Autodesk Inventor part; units mm, degrees
ref_plane "YZ Plane" through (0, 0, 0) normal (1, 0, 0) x (0, 1, 0)
ref_plane "XZ Plane" through (0, 0, 0) normal (0, 1, 0) x (-1, 0, 0)
ref_plane "XY Plane" through (0, 0, 0) normal (0, 0, 1) x (1, 0, 0)
sketch "Эскиз1" plane through (0, 0, 0) normal (0, 0, 1) x (1, 0, 0)
  circle A0 centre (0, 0) radius 11.3
  circle A1 centre (-7.7068, -2.1459) radius 1.55
  circle A2 centre (1.995, 7.7473) radius 1.55
  circle A3 centre (-7.7068, -2.1459) radius 1.55
  circle A4 centre (1.995, 7.7473) radius 1.55
  circle A5 centre (5.7118, -5.6014) radius 1.55
  circle A6 centre (0, 0) radius 11.3
  circle A7 centre (7.7568, 1.9574) radius 2
  circle A8 centre (-2.1832, -7.6963) radius 2
  circle A9 centre (-5.5736, 5.7389) radius 2
  circle A10 centre (0, 0) radius 11.1
  point P0 (0, 0)
extrude "Выдавливание1" add sketch "Эскиз1" along normal blind 5 contours A7 | A8 | A9 | A10
sketch "Эскиз2" plane through (0, 0, 0) normal (0, 0, -1) x (-1, 0, 0)
  circle A0 centre (5.5736, 5.7389) radius 2
  circle A1 centre (2.1832, -7.6963) radius 2
  circle A2 centre (-7.7568, 1.9574) radius 2
  circle A3 centre (5.5736, 5.7389) radius 1.9
  circle A4 centre (2.1832, -7.6963) radius 1.9
  circle A5 centre (-7.7568, 1.9574) radius 1.9
  point P0 (0, 0)
  dimension "d3" = 0.1
  dimension "d4" = 0.1
  dimension "d5" = 0.1
extrude "Выдавливание2" add sketch "Эскиз2" along normal blind 5 contours A3 | A4 | A5
chamfer "Фаска1" distance 1 angle 45 6 edges at (9.6568, 1.9574, -5) (-3.6736, 5.7389, -5) (-0.2832, -7.6963, -5) (4.1618, -5.6014, 5) (0.445, 7.7473, 5) (-9.2568, -2.1459, 5)
properties part number "ВедущееКолесоВнутр"
Model file for the job. Use its own axes, mm. A direction names the side the tool comes from. Coordinates: 2 decimals unless noted, no trailing zeros. Write each loop counter-clockwise with the first axis right and the second up, starting at its lowest first coordinate (ties: lowest second). Pieces come first, ordered by that corner, then holes. Notation, with made-up numbers: (-24, 76) - (16, 76) arc R38 ccw to (16, 114) - close; hole circle Ø10 at (26, 58.5). An arc over 180 degrees is marked (long way). Write each question's results on one line, items separated by ' | '. Start each with the question number.
1) Flat gauge pins, fed straight in: P1, Ø1.5, axis at x = 8.5, z = 1.5, coming from the +Y side; P2, Ø3, axis at y = -7.5, z = 0, coming from the +X side; P3, Ø6, axis at x = 7.5, y = -9, coming from the -Z side; P4, Ø8, axis at x = 7.5, y = -5, coming from the +Z side. Where does each tip first touch, or does it go through?
2) Mould opens along X. For faces 1 (the face through (6.43, -4.23, 1.97)), 2 (the face through (-3.06, -6.01, -1.97)), 3 (the face through (-6, 6, -5)) say: pulls with the +X half, pulls with the -X half, needs draft (parallel to the pull), parting line crosses it, or undercut.
3) 3-axis set-ups, long thin cutter, end or side, ignore diameter. For faces 4 (the face through (-4.173, 4.455, -1.972)), 5 (the face through (-2, -8, -5)): which of +Z, -Z, +X, -X, +Y, -Y reach the whole face in a straight line?
4) Cut at A-A (z = 2.25). Write the cut outline in (x, y) (3 decimals), then the cut area to 3 significant figures.
5) Probe line 1 along Y through (x, z) = (-0.25, 1.75); line 2 along Z through (x, y) = (-4.5, 3.25); line 3 along Y through (x, z) = (-7.25, -2). List the from-to ranges inside material, lowest first. Write a range as from..to.
6) Cut at B-B (z = -0.75). Write the cut outline in (x, y), then the cut area to 3 significant figures.
Returned:
1) P1: y = 7.95 | P2: x = 9.34 | P3: z = 0 | P4: z = 5
2) face 1: undercut | face 2: parting line crosses it | face 3: needs draft
3) face 4: -Z | face 5: -Z, +X, -X, +Y, -Y
4) outline: circle Ø22.2 at (0, 0); hole circle Ø3.1 at (-7.707, -2.146); hole circle Ø3.1 at (1.995, 7.747); hole circle Ø3.1 at (5.712, -5.601) | area: 364 mm^2
5) line 1: -11.1..11.1 | line 2: 0..5 | line 3: 4.84..6.63
6) outline: circle Ø3.8 at (-5.57, 5.74); circle Ø3.8 at (-2.18, -7.7); circle Ø3.8 at (7.76, 1.96) | area: 34.0 mm^2
